from build123d import *

# Parameters (mm, degrees)
SKETCH_W        = 92.210236
SKETCH_H        = 26
PAD_DEPTH       = 10
SKETCH001_W     = 8.9
SKETCH001_H     = 10
PAD001_DEPTH    = 8.95
CHAMFER_SIZE    = 0.5
CHAMFER001_SIZE = 0.5
SKETCH002_W     = 8.9
SKETCH002_H     = 10
PAD002_DEPTH    = 8.95
CHAMFER002_SIZE = 0.5
CHAMFER003_SIZE = 0.5
FILLET_R        = 1.95
FILLET001_R     = 1.95


with BuildPart() as part:
    # Sketch → Pad (new body)
    with BuildSketch(Plane.XZ):
        Rectangle(SKETCH_W, SKETCH_H)
        Polygon((-44.105118, 11), (-44.105118, -11), (-31.403412, -11), align=None, mode=Mode.SUBTRACT)
        Polygon((-29.403412, -11), (-42.105118, 11), (-16.701706, 11), align=None, mode=Mode.SUBTRACT)
        Polygon((-14.701706, 11), (-27.403412, -11), (-2, -11), align=None, mode=Mode.SUBTRACT)
        Polygon((-12.701706, 11), (12.701706, 11), (0, -11), align=None, mode=Mode.SUBTRACT)
        Polygon((14.701706, 11), (2, -11), (27.403412, -11), align=None, mode=Mode.SUBTRACT)
        Polygon((16.701706, 11), (42.105118, 11), (29.403412, -11), align=None, mode=Mode.SUBTRACT)
        Polygon((44.105118, 11), (44.105118, -11), (31.403412, -11), align=None, mode=Mode.SUBTRACT)
    extrude(amount=PAD_DEPTH)

    # Sketch001 (on Face4 of Pad) → Pad001 (join)
    with BuildSketch(Plane(origin=(-46.105118, 0, 0), x_dir=(0, 0, -1), z_dir=(-1, 0, 0))):
        with Locations((0, 5)):
            Rectangle(SKETCH001_W, SKETCH001_H)
    extrude(amount=PAD001_DEPTH)

    # Chamfer
    chamfer_edges = [part.edges().sort_by_distance(p)[0] for p in [
        (-55.055118, -5, 4.45),
    ]]
    chamfer(chamfer_edges, length=CHAMFER_SIZE)

    # Chamfer001
    chamfer001_edges = [part.edges().sort_by_distance(p)[0] for p in [
        (-55.055118, -5, -4.45),
    ]]
    chamfer(chamfer001_edges, length=CHAMFER001_SIZE)

    # Sketch002 (on Face12 of Chamfer001) → Pad002 (join)
    with BuildSketch(Plane(origin=(46.105118, 0, 0), x_dir=(0, 0, 1), z_dir=(1, 0, 0))):
        with Locations((0, 5)):
            Rectangle(SKETCH002_W, SKETCH002_H)
    extrude(amount=PAD002_DEPTH)

    # Chamfer002
    chamfer002_edges = [part.edges().sort_by_distance(p)[0] for p in [
        (55.055118, -5, 4.45),
    ]]
    chamfer(chamfer002_edges, length=CHAMFER002_SIZE)

    # Chamfer003
    chamfer003_edges = [part.edges().sort_by_distance(p)[0] for p in [
        (55.055118, -5, -4.45),
    ]]
    chamfer(chamfer003_edges, length=CHAMFER003_SIZE)

    # Fillet
    fillet_edges = [part.edges().sort_by_distance(p)[0] for p in [
        (0, 0, 13),
    ]]
    fillet(fillet_edges, radius=FILLET_R)

    # Fillet001
    fillet001_edges = [part.edges().sort_by_distance(p)[0] for p in [
        (0, 0, -13),
    ]]
    fillet(fillet001_edges, radius=FILLET001_R)


solid = part.part
The listing builds one solid part. Answer for the finished solid, in the listing's coordinates (mm). A direction names the side the tool comes from. Coordinates: 2 decimals unless noted, no trailing zeros. Order: outer loops, then holes, each group sorted by start corner. A loop starts at its lowest first (then second) coordinate and runs counter-clockwise, first axis right, second up.
Q1. Which of the six approach directions +Z, -Z, +X, -X, +Y, -Y give full straight-line access (tool end or side, diameter ignored) to faces 1 (the face through (46.105, -5, 9)), 2 (the face through (-50, -5, 4.45)), 3 (the face through (38, -5, -11))?
Q2. Consider line 1 (Z direction, x = 35.5, y = -9.5); line 2 (Z direction, x = 12, y = -9); line 3 (Y direction, x = -17, z = 11.25). Determine where each line is inside the solid, lowest interval first.
Q3. For a pull along Z with two mould halves and no side action, classify faces 4 (the face through (29, -5, 11)), 5 (the face through (46.105, -5, -9)), 6 (the face through (-1, -6, -13)) as pulls with the +Z half, pulls with the -Z half, needs draft (parallel to the pull), parting line crosses it, or undercut.
Q4. A cutting plane is placed at B-B, the plane z = 6. State how many separate pieces and enclosed holes the cut face has, and give its area (3 significant figures).
Q5. Given P1, Ø4.5, axis at y = -5.5, z = 10, coming from the +X side; P2, Ø2.5, axis at x = -49.5, y = -3, coming from the -Z side; P3, Ø2.5, axis at y = -4.5, z = 11, coming from the -X side, each flat-ended and moving along its own axis, determine where each tip first touches the part or whether it passes through.
Q6. A cutting plane is placed at A-A, the plane x = -23. Write down the section's boundary in (y, z).
Q7. A cutting plane is placed at D-D, the plane x = 47.5. Write down the section's boundary in (y, z).
Answers follow:
1. face 1: +Z, +X, +Y, -Y
1. face 2: +Z, -X, +Y, -Y
1. face 3: +Y, -Y
2. line 1: z = -13 to -11, -3.9 to -0.44, 11 to 13
2. line 2: z = -13 to -11, 6.32 to 9.78, 11 to 13
2. line 3: y = -10 to -0.01
3. face 4: undercut
3. face 5: needs draft
3. face 6: pulls with the -Z half
4. separate pieces: 8
4. enclosed holes: 0
4. area: 160 mm2
5. P1: stops at x = 46.11
5. P2: stops at z = -4.45
5. P3: stops at x = -46.11
6. outline: (-10, -13) - (-1.95, -13) arc R1.95 ccw to (0, -11.05) - (0, -11) - (-10, -11) - close; (-10, -3.37) - (0, -3.37) - (0, 0.09) - (-10, 0.09) - close; (-10, 11) - (0, 11) - (0, 11.05) arc R1.95 ccw to (-1.95, 13) - (-10, 13) - close
7. outline: (-10, -4.45) - (0, -4.45) - (0, 4.45) - (-10, 4.45) - close
